```python
from build123d import *

# Parameters (mm, degrees)
CROQUIS1_R              = 1.75
CROQUIS1_R_2            = 1.65
SALIENTE_EXTRUIR1_DEPTH = 89.8
CROQUIS2_W              = 6.07
CROQUIS2_H              = 7
CORTAR_EXTRUIR1_DEPTH   = 138.205284155


with BuildPart() as part:
    # Croquis1 → Saliente-Extruir1 (new body)
    with BuildSketch(Plane.XY):
        with BuildLine():
            Line((-3.5, 100), (-3.5, -15))
            ThreePointArc((-3.5, -15), (0, -18.5), (3.5, -15))
            Line((3.5, -15), (3.5, 100))
            ThreePointArc((3.5, 100), (0, 103.5), (-3.5, 100))
        make_face()
        Circle(CROQUIS1_R, mode=Mode.SUBTRACT)
        with Locations((0, -15)):
            Circle(CROQUIS1_R, mode=Mode.SUBTRACT)
        with Locations((0, 100)):
            Circle(CROQUIS1_R_2, mode=Mode.SUBTRACT)
    extrude(amount=-SALIENTE_EXTRUIR1_DEPTH)

    # Croquis2 → Cortar-Extruir1 (cut, through all)
    with BuildSketch(Plane(origin=(3.5, 0, 0), x_dir=(0, 0, -1), z_dir=(1, 0, 0))):
        Polygon((2, 4), (2, -18.5), (87.8, -18.5), (87.8, 4), (85.8, 4), (85.8, 34), (58.253185901, 91.58113315), (31.546814099, 91.58113315), (4, 34), (4, 4), align=None)
        with Locations((44.9, 100)):
            Rectangle(CROQUIS2_W, CROQUIS2_H)
        Polygon((0, 34), (29.9, 96.5), (35.97, 96.5), (35.97, 103.5), (0, 103.5), align=None)
        Polygon((59.9, 96.5), (89.8, 34), (89.8, 103.5), (53.83, 103.5), (53.83, 96.5), align=None)
    extrude(amount=-CORTAR_EXTRUIR1_DEPTH, mode=Mode.SUBTRACT)


solid = part.part
```
Geometry check sheet. Reference: the model listing, model coordinates, mm. A direction names the side the tool comes from. Round coordinates to 2 decimals unless told otherwise and drop trailing zeros. Order: outer loops, then holes, each group sorted by start corner. A loop starts at its lowest first (then second) coordinate and runs counter-clockwise, first axis right, second up. Notation, with made-up numbers: (39.25, 87.5) -> (89.25, 87.5) arc R24 ccw to (89.25, 101.5) -> close; hole circle Ø10 at (38, 33). An arc over 180 degrees is marked (long way). Return JSON: item names as keys, results as strings. Group by question number.
Q1. Material ranges on probe 1 along X at (y, z) = (100, -40.35); probe 2 along Z at (x, y) = (3, 29); probe 3 along Y at (x, z) = (0, -51.75), recorded low to high. Write a range as from..to.
Q2. Section check A-A, the plane y = 0. Record the boundary of the cut face in (x, z), plus the area to 3 significant figures.
Q3. Tool access check on faces 4 (the flat face through (0.049, 63.194, -17.966)), 5 (the flat face through (0, 96.5, -33)), 6 (the flat face through (0, 96.5, -45)). Record the directions out of +Z, -Z, +X, -X, +Y, -Y that give a thin tool (end or side, any length) a straight path to the whole face; none if there is none.
Q4. Section check B-B, the plane y = 89. Record the boundary of the cut face in (x, z), plus the area to 3 significant figures.
Q5. Section check D-D, the plane z = -64. Record the boundary of the cut face in (x, y), plus the area to 3 significant figures.
Q6. Section check C-C, the plane x = 0. Count the separate pieces of the cut face and the enclosed holes in it, plus the area to 3 significant figures.
Q7. Release check for a two-part mould opening along Z. For faces 1 (the flat face through (0.05, 65.69, -74.64)), 2 (the cylindrical face through (-0.228, -13.265, -0.986)), 3 (the flat face through (0, 19, -85.8)) record: released by +Z, released by -Z, zero draft, split by the parting line, or undercut.
Q8. Gauge pin test, flat ends, axial feed: pin 1 (1.6 mm diameter, centred on x = 1.5, z = -3, fed in from -Y); pin 2 (3.5 mm diameter, centred on x = 1.5, y = 101, fed in from -Z); pin 3 (4 mm diameter, centred on x = 1, y = 85, fed in from +Z). Record the tip position at first contact, or that the pin passes through.
Numbers:
{
 "1": {"probe 1": "-3.5..-1.65, 1.65..3.5", "probe 2": "-89.8..-85.8, -4..0", "probe 3": "91.58..98.35, 101.65..103.5"},
 "2": {"outline": "(-3.5, -89.8) -> (-1.75, -89.8) -> (-1.75, -87.8) -> (-3.5, -87.8) -> close; (-3.5, -2) -> (-1.75, -2) -> (-1.75, 0) -> (-3.5, 0) -> close; (1.75, -89.8) -> (3.5, -89.8) -> (3.5, -87.8) -> (1.75, -87.8) -> close; (1.75, -2) -> (3.5, -2) -> (3.5, 0) -> (1.75, 0) -> close", "area": "14.0 mm^2"},
 "3": {"face 4": "+X, -X, -Y", "face 5": "+Z, +X, -X, +Y", "face 6": "+X, -X, +Y"},
 "4": {"outline": "(-3.5, -63.49) -> (3.5, -63.49) -> (3.5, -59.49) -> (-3.5, -59.49) -> close; (-3.5, -30.31) -> (3.5, -30.31) -> (3.5, -26.31) -> (-3.5, -26.31) -> close", "area": "56.0 mm^2"},
 "5": {"outline": "(-3.5, 79.57) -> (3.5, 79.57) -> (3.5, 87.93) -> (-3.5, 87.93) -> close", "area": "58.5 mm^2"},
 "6": {"separate pieces": "7", "enclosed holes": "0", "area": "965 mm^2"},
 "7": {"face 1": "released by -Z", "face 2": "zero draft", "face 3": "undercut"},
 "8": {"pin 1": "y = 4", "pin 2": "z = -53.83", "pin 3": "z = -23.44"}
}
